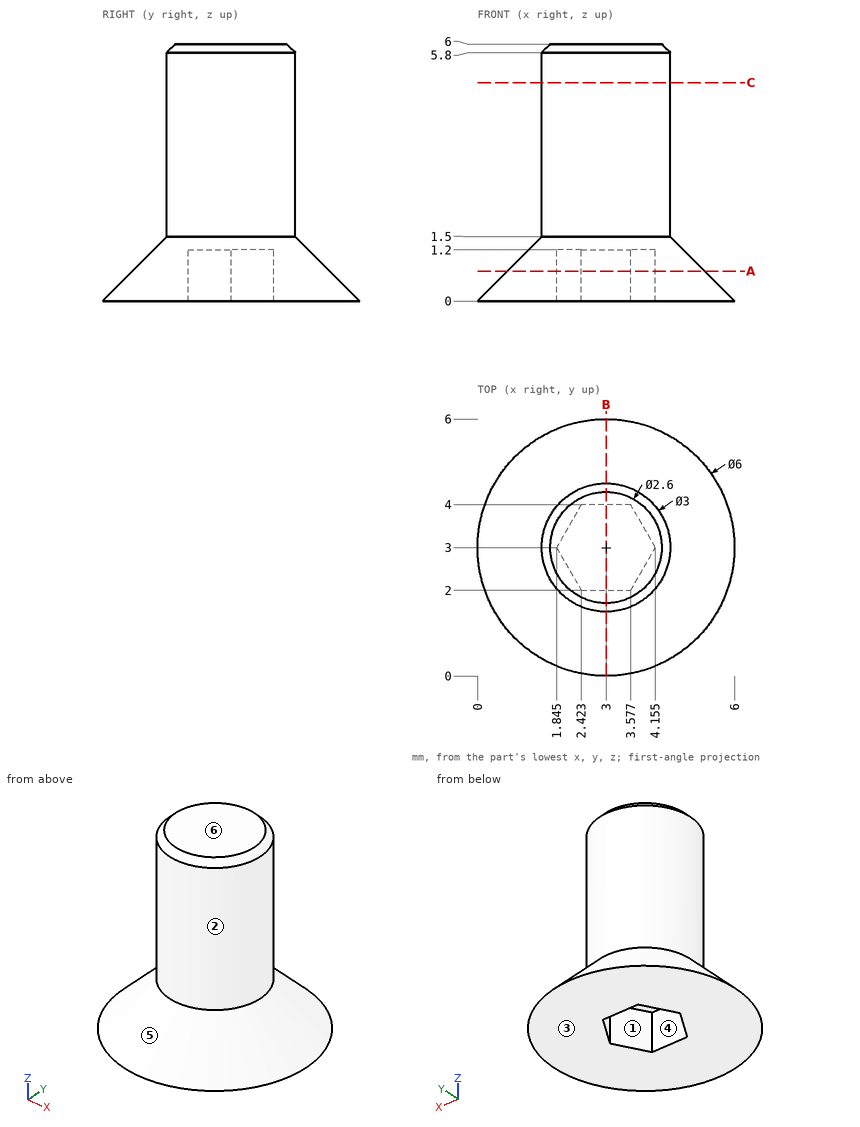
Design review of the part shown in the three views and the two pictorial views. Dimensions are in mm from the part's minimum x, y and z. A direction names the side the tool comes from. Coordinates: 2 decimals unless noted, no trailing zeros. Order: outer loops, then holes, each group sorted by start corner. A loop starts at its lowest first (then second) coordinate and runs counter-clockwise, first axis right, second up.
Item 1: For line 1 (Z direction, x = 3.7, y = 3.25); line 2 (X direction, y = 4.1, z = 2.7); line 3 (Y direction, x = 3.55, z = 3.5) (1 decimal), list the stretches that pass through material, from the lowest coordinate up.
Item 2: For pin 1 Ø2 at (x, y) = (5.5, 1) entering from +Z; pin 2 Ø0.6 at (x, z) = (3, 1) entering from -Y; pin 3 Ø3 at (y, z) = (5, 3.5) entering from -X (1 decimal), all flat-tipped, find the tip position at first contact; note any pin that passes through.
Item 3: Take a section at B-B, the plane x = 3. Write out the cut boundary in (y, z).
Item 4: Take a section at A-A, the plane z = 0.7. Write out the cut boundary in (x, y) (1 decimal).
Item 5: The part is to be moulded in two halves that separate along Y. For the marked faces 4, 5 and 6, say which applies: pulls with the +Y half, pulls with the -Y half, needs draft (parallel to the pull), parting line crosses it, or undercut.
Item 6: For the marked faces 1, 2 and 3, list the 3-axis set-ups (+Z, -Z, +X, -X, +Y, -Y) from which the entire face can be reached by the end or side of a thin tool; tool diameter is ignored.
Item 7: Take a section at C-C, the plane z = 5.1. Write out the cut boundary in (x, y).
The answers:
1. line 1: z = 1.2 to 6
1. line 2: x = 1.98 to 4.02
1. line 3: y = 1.6 to 4.4
2. pin 1: stops at z = 0.8
2. pin 2: stops at y = 0.7
2. pin 3: stops at x = 1.6
3. outline: (0, 0) - (2, 0) - (2, 1.2) - (4, 1.2) - (4, 0) - (6, 0) - (4.5, 1.5) - (4.5, 5.8) - (4.3, 6) - (1.7, 6) - (1.5, 5.8) - (1.5, 1.5) - close
4. outline: circle Ø4.6 at (3, 3); hole (1.8, 3) - (2.4, 2) - (3.6, 2) - (4.2, 3) - (3.6, 4) - (2.4, 4) - close
5. face 4: undercut
5. face 5: parting line crosses it
5. face 6: needs draft
6. face 1: -Z
6. face 2: +Z
6. face 3: -Z, +X, -X, +Y, -Y
7. outline: circle Ø3 at (3, 3)
